Can you work these out from the model? Positions are in its coordinate system, mm. Face numbers are marked on the shaded views. A direction names the side the tool comes from. Give positions to 0.01 mm unless a question says otherwise; leave off trailing zeros. Use a Markdown table: item, result. Add a question column.
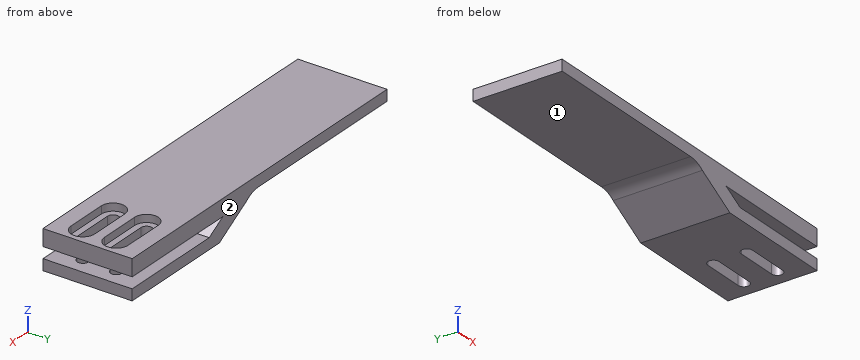
```python
from build123d import *

# Parameters (mm, degrees)
BOSS_EXTRUDE1_DEPTH = 25.4
SKETCH3_W           = 55.88
SKETCH3_H           = 25.4
CUT_EXTRUDE1_DEPTH  = 1.5875
FILLET1_R           = 7.62
CUT_EXTRUDE2_REACH  = 107.315
CUT_EXTRUDE3_DEPTH  = 2.159


with BuildPart() as part:
    # Sketch1 → Boss-Extrude1 (new body)
    with BuildSketch(Plane(origin=(0, 0, 0), x_dir=(1, 0, 0), z_dir=(0, 1, 0))):
        Polygon((-22.587652327, -6.35), (-36.195, -6.35), (-30.695738686, -3.175), (-15.498938433, -3.175), (0, -3.175), (0, 0), (-34.721477372, 0), (-45.72, -6.35), (-101.6, -6.35), (-101.6, -11.1125), (0, -11.1125), (0, -6.35), (-15.498938433, -6.35), align=None)
    extrude(amount=BOSS_EXTRUDE1_DEPTH)

    # Sketch3 → Cut-Extrude1 (cut)
    with BuildSketch(Plane(origin=(0, 0, 6.35), x_dir=(-1, 0, 0), z_dir=(0, 0, -1))):
        with Locations((73.66, 12.7)):
            Rectangle(SKETCH3_W, SKETCH3_H)
    extrude(amount=-CUT_EXTRUDE1_DEPTH, mode=Mode.SUBTRACT)

    # Fillet1
    # the kernel refuses this fillet: 7.62 mm, written as the material it adds along each edge
    with BuildSketch(Plane(origin=(-45.72, 0, 7.9375), x_dir=(-1, 0, 0), z_dir=(0, 1, 0))) as fillet1_piece_1:
        with BuildLine():
            CenterArc((4.65546386, -7.62), FILLET1_R, 90, 37.658462006)
            Line((0, -1.5875), (-0.093109277, -1.46685))
            ThreePointArc((-0.093109277, -1.46685), (-0.1524, -0.79375), (-0.1524, 0))
            Line((-0.1524, 0), (0, 0.1524))
            Line((0, 0.1524), (4.65546386, 0.1524))
            Line((4.65546386, 0.1524), (4.65546386, 0))
        make_face()
    extrude(amount=25.4)

    # Cut-Extrude2: up to this face of the body (flat: up to its plane)
    cut_extrude2_end = Plane(part.part.faces().sort_by_distance((-17.360738686, 12.7, 0))[0])
    # Sketch4 → Cut-Extrude2 (cut, up to the picked face)
    with BuildSketch(Plane.XY.offset(11.1125), mode=Mode.PRIVATE) as cut_extrude2_sk1:
        with BuildLine():
            Line((-4.7625, 19.05), (-16.8275, 19.05))
            ThreePointArc((-16.8275, 19.05), (-18.415, 17.4625), (-16.8275, 15.875))
            Line((-16.8275, 15.875), (-4.7625, 15.875))
            ThreePointArc((-4.7625, 15.875), (-3.175, 17.4625), (-4.7625, 19.05))
        make_face()
    cut_extrude2_tool1 = split(extrude(cut_extrude2_sk1.sketch, amount=-CUT_EXTRUDE2_REACH, mode=Mode.PRIVATE), bisect_by=cut_extrude2_end, keep=Keep.BOTH, mode=Mode.PRIVATE)
    # Sketch4 → Cut-Extrude2 (cut, up to the picked face)
    with BuildSketch(Plane.XY.offset(11.1125), mode=Mode.PRIVATE) as cut_extrude2_sk2:
        with BuildLine():
            Line((-4.7625, 6.35), (-16.8275, 6.35))
            ThreePointArc((-16.8275, 6.35), (-18.415, 7.9375), (-16.8275, 9.525))
            Line((-16.8275, 9.525), (-4.7625, 9.525))
            ThreePointArc((-4.7625, 9.525), (-3.175, 7.9375), (-4.7625, 6.35))
        make_face()
    cut_extrude2_tool2 = split(extrude(cut_extrude2_sk2.sketch, amount=-CUT_EXTRUDE2_REACH, mode=Mode.PRIVATE), bisect_by=cut_extrude2_end, keep=Keep.BOTH, mode=Mode.PRIVATE)
    add(cut_extrude2_tool1.solids().sort_by(Axis((-10.795, 17.4625, 11.1125), (0, 0, -1)))[0], mode=Mode.SUBTRACT)
    add(cut_extrude2_tool2.solids().sort_by(Axis((-10.795, 7.9375, 11.1125), (0, 0, -1)))[0], mode=Mode.SUBTRACT)

    # Sketch5 → Cut-Extrude3 (cut)
    with BuildSketch(Plane.XY.offset(11.1125)):
        with BuildLine():
            Line((-4.7625, 4.572), (-16.8275, 4.572))
            ThreePointArc((-16.8275, 4.572), (-20.193, 7.9375), (-16.8275, 11.303))
            Line((-16.8275, 11.303), (-4.7625, 11.303))
            ThreePointArc((-4.7625, 11.303), (-1.397, 7.9375), (-4.7625, 4.572))
        make_face()
        with BuildLine():
            Line((-4.7625, 14.097), (-16.8275, 14.097))
            ThreePointArc((-16.8275, 14.097), (-20.193, 17.4625), (-16.8275, 20.828))
            Line((-16.8275, 20.828), (-4.7625, 20.828))
            ThreePointArc((-4.7625, 20.828), (-1.397, 17.4625), (-4.7625, 14.097))
        make_face()
    extrude(amount=-CUT_EXTRUDE3_DEPTH, mode=Mode.SUBTRACT)


solid = part.part
```
1. Will these pins go through, and if not, where does the flat tip stop? P1, Ø12.5, axis at x = -12.5, y = 10.5, coming from the +Z side; P2, Ø1.5, axis at x = -28.5, z = 4.5, coming from the +Y side.
2. Suppose I cut it at A-A (x = -15). State how many separate pieces and enclosed holes the cut face has, and give its area (3 significant figures).
3. Please list where these lines run through material, in increasing order: line 1 along X through (y, z) = (8.25, 7); line 2 along Z through (x, y) = (-70, 24.5); line 3 along X through (y, z) = (17.75, 1.75). Write a range as [from, to].
4. On a 3-axis mill with a long thin cutter (end or side, diameter ignored), from which of +Z, -Z, +X, -X, +Y, -Y can I reach the whole of each face in a straight line? I mean the marked faces 1 and 2. Say none if no direction works.
Results below:
| question | item | result |
|---|---|---|
| 1 | P1 | z = 11.11 |
| 1 | P2 | through |
| 2 | separate pieces | 6 |
| 2 | enclosed holes | 0 |
| 2 | area | 136 mm² |
| 3 | line 1 | [-46.71, -18.38], [-3.21, 0] |
| 3 | line 2 | [7.94, 11.11] |
| 3 | line 3 | [-37.75, -18.39], [-3.2, 0] |
| 4 | face 1 | -Z, -X, +Y, -Y |
| 4 | face 2 | +Z, -Z, +X, -X, +Y |
